Autodesk Inventor part; units mm, degrees
ref_plane "C1_XY" through (0, 0, 0) normal (0, 0, 1) x (1, 0, 0)
ref_plane "C1_YZ" through (0, 0, 0) normal (1, 0, 0) x (0, 1, 0)
ref_plane "C1_ZX" through (0, 0, 0) normal (0, 1, 0) x (0, 0, 1)
sketch "Sketch_122" plane through (0, 0, 0) normal (0, 0, 1) x (1, 0, 0)
  arc A0 (-15, -13) -> (-13, -15) centre (-13, -13) ccw
  line L0 (-13, -15) -> (13, -15)
  arc A1 (13, -15) -> (15, -13) centre (13, -13) ccw
  line L1 (15, -13) -> (15, 13)
  arc A2 (15, 13) -> (13, 15) centre (13, 13) ccw
  line L2 (13, 15) -> (-13, 15)
  arc A3 (-13, 15) -> (-15, 13) centre (-13, 13) ccw
  line L3 (-15, 13) -> (-15, 4)
  line L4 (-15, 4) -> (-13, 4)
  line L5 (-13, 4) -> (-13, 8.25)
  line L6 (-13, 8.25) -> (-9.6642, 8.25)
  line L7 (-9.6642, 8.25) -> (-6, 4.5858)
  line L8 (-6, 4.5858) -> (-6, 0.5196)
  line L9 (-6, 0.5196) -> (-5.7, 0)
  line L10 (-5.7, 0) -> (-6, -0.5196)
  line L11 (-6, -0.5196) -> (-6, -4.5858)
  line L12 (-6, -4.5858) -> (-9.6642, -8.25)
  line L13 (-9.6642, -8.25) -> (-13, -8.25)
  line L14 (-13, -8.25) -> (-13, -4)
  line L15 (-13, -4) -> (-15, -4)
  line L16 (-15, -4) -> (-15, -13)
  line L17 (6, -4.5858) -> (9.6642, -8.25)
  line L18 (9.6642, -8.25) -> (13, -8.25)
  line L19 (13, -8.25) -> (13, 8.25)
  line L20 (13, 8.25) -> (9.6642, 8.25)
  line L21 (9.6642, 8.25) -> (6, 4.5858)
  line L22 (6, 4.5858) -> (6, -4.5858)
extrude "Extrusion1" add sketch "Sketch_122" against normal blind 417
sketch "Sketch2" plane through (0, 0, -417) normal (0, 0, -1) x (-1, 0, 0)
  point P0 (0, 0)
hole "Hole1" at (0, 0, -417) direction (0, 0, 1) diameter 6.8 depth 600
sketch "Sketch_173" plane through (0, 0, 0) normal (0, 0, 1) x (1, 0, 0)
  arc A0 (-9.8177, 12.6944) -> (-11.625, 9.525) centre (-11.625, 11.625) ccw
  line L0 (-11.625, 9.525) -> (-8.1108, 9.525)
  line L1 (-8.1108, 9.525) -> (-4.5858, 6)
  line L2 (-4.5858, 6) -> (4.5858, 6)
  line L3 (4.5858, 6) -> (8.1108, 9.525)
  line L4 (8.1108, 9.525) -> (11.625, 9.525)
  arc A1 (11.625, 9.525) -> (9.8177, 12.6944) centre (11.625, 11.625) ccw
  arc A2 (8.7013, 13) -> (9.8177, 12.6944) centre (9.3013, 13) ccw
  line L5 (8.7013, 13) -> (-8.7013, 13)
  arc A3 (-9.8177, 12.6944) -> (-8.7013, 13) centre (-9.3013, 13) ccw
extrude "Extrusion2" cut sketch "Sketch_173" against normal blind 600
sketch "Sketch_174" plane through (0, 0, 0) normal (0, 0, 1) x (1, 0, 0)
  arc A0 (-11.625, -9.525) -> (-9.8177, -12.6944) centre (-11.625, -11.625) ccw
  arc A1 (-8.7013, -13) -> (-9.8177, -12.6944) centre (-9.3013, -13) ccw
  line L0 (-8.7013, -13) -> (8.7013, -13)
  arc A2 (9.8177, -12.6944) -> (8.7013, -13) centre (9.3013, -13) ccw
  arc A3 (9.8177, -12.6944) -> (11.625, -9.525) centre (11.625, -11.625) ccw
  line L1 (11.625, -9.525) -> (8.1108, -9.525)
  line L2 (8.1108, -9.525) -> (4.5858, -6)
  line L3 (4.5858, -6) -> (-4.5858, -6)
  line L4 (-4.5858, -6) -> (-8.1108, -9.525)
  line L5 (-8.1108, -9.525) -> (-11.625, -9.525)
extrude "Extrusion3" cut sketch "Sketch_174" against normal blind 600
ref_plane "C1_XY" through (0, 0, 0) normal (0, 0, 1) x (1, 0, 0)
ref_plane "C1_YZ" through (0, 0, 0) normal (1, 0, 0) x (0, 1, 0)
ref_plane "C1_ZX" through (0, 0, 0) normal (0, 1, 0) x (0, 0, 1)
ref_plane "to_frame_cap1_XY" through (0, 0, 0) normal (0, 0, 1) x (1, 0, 0)
ref_plane "to_frame_cap1_YZ" through (0, 0, 0) normal (1, 0, 0) x (0, 1, 0)
ref_plane "to_frame_cap1_ZX" through (0, 0, 0) normal (0, 1, 0) x (0, 0, 1)
ref_plane "to_frame_cap2_XY" through (0, 0, -600) normal (0, 0, -1) x (1, 0, 0)
ref_plane "to_frame_cap2_YZ" through (0, 0, -600) normal (1, 0, 0) x (0, -1, 0)
ref_plane "to_frame_cap2_ZX" through (0, 0, -600) normal (0, -1, 0) x (0, 0, -1)
thread "Thread1"
thread "Thread2"
properties part number "HFSC6-3030-417" material "Aluminum 6061"
Design review of the part built by this model. Coordinates are the model's own, in mm. A direction names the side the tool comes from. Give positions to 0.01 mm unless a question says otherwise; leave off trailing zeros. Order: outer loops, then holes, each group sorted by start corner. A loop starts at its lowest first (then second) coordinate and runs counter-clockwise, first axis right, second up. Notation, with made-up numbers: (81, -39.5) - (123, -39.5) arc R21 ccw to (123, -10.5) - close; hole circle Ø2 at (-39, 6.25). An arc over 180 degrees is marked (long way). Use a Markdown table: item, result. Add a question column.
(1) Add section A-A on x = 0. Give the boundary of the cut face in (y, z).
(2) Machinability: for faces 5 (the face through (0, 6, -206)), 6 (the face through (0, -15, -206)), which of the approach directions +Z, -Z, +X, -X, +Y, -Y give a long, thin tool a straight path to every point of the face, cutting with its end or side? Answer none if there is none.
(3) Clearance check with flat-ended pins moving along their axes: P1, Ø8, axis at x = -6, y = -11.5, coming from the +Z side; P2, Ø1.6, axis at x = -14, z = -105.5, coming from the +Y side. State where each tip first meets the part, or that it passes through.
(4) Add section B-B on z = -367.5. Give the number of separate pieces and of enclosed holes in the cut face, then the cut area to 3 significant figures.
(5) Mouldability with a two-part tool opening along X and no side actions: class faces 1 (the face through (0, 13, -206)), 2 (the face through (-15, -8, -206)), 3 (the face through (3.32, -0.74, -205.58)), 4 (the face through (0, 4, -417)) as +X half, -X half, draft (parallel to the pull), parting line (faces both ways), or undercut.
(6) Wall thickness on probe 1 along Y at (x, z) = (-12, -181); probe 2 along Y at (x, z) = (0, -142); probe 3 along Y at (x, z) = (3.75, -322.5): over which ranges is each line inside the solid? List them lowest first. Write a range as [from, to].
Report:
| question | item | result |
|---|---|---|
| 1 | outline | (-15, -417) - (-13, -417) - (-13, 0) - (-15, 0) - close; (-6, -417) - (-3.4, -417) - (-3.4, 0) - (-6, 0) - close; (3.4, -417) - (6, -417) - (6, 0) - (3.4, 0) - close; (13, -417) - (15, -417) - (15, 0) - (13, 0) - close |
| 2 | face 5 | +Z, -Z |
| 2 | face 6 | +Z, -Z, +X, -X, -Y |
| 3 | P1 | stops at z = 0 |
| 3 | P2 | stops at y = 14.99 |
| 4 | separate pieces | 1 |
| 4 | enclosed holes | 4 |
| 4 | area | 360 mm² |
| 5 | face 1 | undercut |
| 5 | face 2 | -X half |
| 5 | face 3 | undercut |
| 5 | face 4 | draft |
| 6 | probe 1 | y = [-15, -13.69], [-9.56, -8.25], [8.25, 9.56], [13.69, 15] |
| 6 | probe 2 | y = [-15, -13], [-6, -3.4], [3.4, 6], [13, 15] |
| 6 | probe 3 | y = [-15, -13], [-6, 6], [13, 15] |
